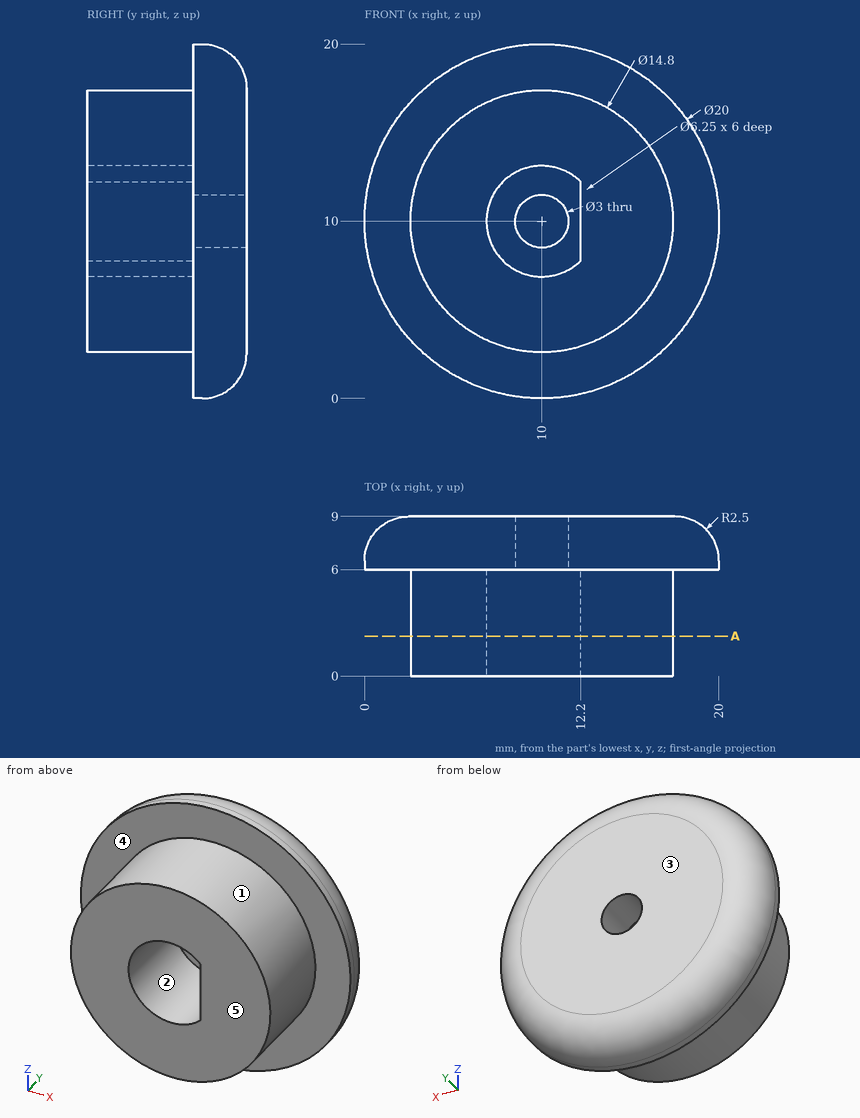
Can you work these out from the drawing? Everything is in mm from the part's minimum corner. A direction names the side the tool comes from. Round coordinates to 2 decimals unless told otherwise and drop trailing zeros. Loops run counter-clockwise (first coordinate to the right, second up) from the corner with the lowest first, then second, coordinate; pieces in that order, holes last.
1. For P1, Ø3, axis at y = 3.5, z = 12, coming from the -X side; P2, Ø4, axis at x = 7, y = 2.5, coming from the +Z side; P3, Ø1.6, axis at x = 10.5, z = 11, coming from the -Y side, each with a flat end and sliding along its axis, tell me the tip position at first contact or that it passes through.
Answer list:
P1: stops at x = 2.62
P2: stops at z = 17.33
P3: stops at y = 6
2. If we section it at A-A on y = 2.25: Write out the boundary of the cut face in (x, z) (3 decimals), plus the area to 3 significant figures.
Answer list:
outline: circle Ø14.8 at (10, 10); hole (12.2, 7.781) - (12.2, 12.219) arc R3.125 ccw (long way) to start
area: 144 mm2
3. Which directions (+Z, -Z, +X, -X, +Y, -Y) give clear straight access to the entire face, cutting with the end or side of a thin tool? Please do the marked faces 4 and 5.
Answer list:
face 4: -Y
face 5: +Z, -Z, +X, -X, -Y
4. If I drill on line 1 along X through (y, z) = (5, 8.25); line 2 along X through (y, z) = (6.7, 10); line 3 along Z through (x, y) = (8, 1), over which ranges is the centre line in solid material (lowest first)?
Answer list:
line 1: x = 2.81 to 7.41, 12.2 to 17.19
line 2: x = 0.01 to 8.5, 11.5 to 19.99
line 3: z = 2.88 to 7.6, 12.4 to 17.12
5. We'd pull the mould along X, two halves only. Please class the marked faces 1, 2 and 3: +X half, -X half, draft (parallel to the pull), parting line (faces both ways), or undercut.
Answer list:
face 1: parting line
face 2: undercut
face 3: draft
